Here's how the part is built. I have some questions about the finished solid (model axes, mm). A direction names the side the tool comes from. Give positions to 0.01 mm unless a question says otherwise; leave off trailing zeros. Order: outer loops, then holes, each group sorted by start corner. A loop starts at its lowest first (then second) coordinate and runs counter-clockwise, first axis right, second up. Notation, with made-up numbers: M -19,-2 L 35,-2 A15 ccw 35,24 Z; hole C 46,15 d7. An arc over 180 degrees is marked long. Use one line per item in the form item = value.
from build123d import *

# Parameters (mm, degrees)
F0_W        = 50.8
F0_H        = 50.8
F1_DEPTH    = 6.35
F3_DEPTH    = 9.144
F2_R        = 6.7603485979
F4_DEPTH    = 25.4
F5_R        = 5.08
F6_T1_DEPTH = 86.0732038629
F7_T        = 2.54
F7_T4_ANGLE = 49.6458001059
F7_T6_ANGLE = 79.2883730852


# Not quite as in the source:
# - a fillet or chamfer that OpenCascade refuses, or shapes differently, is made with other operations: its cross-section is extruded or revolved along the edge and cut away or added
# - a shell that OpenCascade refuses in one call is made with other operations: the cavity is built on its own and cut out


with BuildPart() as f1:
    # F0 (on Top) → F1 (new body)
    with BuildSketch(Plane.XY):
        with Locations((-25.4, 25.4)):
            Rectangle(F0_W, F0_H)
    extrude(amount=-F1_DEPTH)

    # F2 (on face) → F3 (join)
    with BuildSketch(Plane(origin=(0, 0, -6.35), x_dir=(1, 0, 0), z_dir=(0, 0, -1))):
        with BuildLine():
            ThreePointArc((0, 0), (-5.5886686099, -15.504363354), (-19.7841264307, -23.8773841411))
            ThreePointArc((-19.7841264307, -23.8773841411), (-12.8545439956, -39.5156757118), (0, -50.8))
            Line((0, -50.8), (0, 0))
        make_face()
    extrude(amount=F3_DEPTH)

    # F2 (on face) → F4 (cut)
    with BuildSketch(Plane(origin=(0, 0, -6.35), x_dir=(1, 0, 0), z_dir=(0, 0, -1))):
        with Locations((-37.9167422652, -20.3997846693)):
            Circle(F2_R)
    extrude(amount=-F4_DEPTH, mode=Mode.SUBTRACT)

    # F5
    f5_edges = [f1.edges().sort_by_distance(p)[0] for p in [
        (-50.8, 25.4, -6.35),
    ]]
    fillet(f5_edges, radius=F5_R)

    # F6: chamfer of 5.08 on 1 edges, made by hand

    # F6_s2 → F6_t1 (cut)
    with BuildSketch(Plane.XZ.offset(-63.8641495789)):
        Polygon((0, -10.414), (-5.08, -15.494), (0, -15.494), align=None)
    extrude(amount=F6_T1_DEPTH, mode=Mode.SUBTRACT)

    # F7: shell of thickness 2.54, made by hand


with BuildPart() as f7_core1:
    # F7_t2: copy of F1
    add(f1.part)

    # the walls: a layer under each face that stays
    f7_faces = [f7_core1.faces().sort_by_distance(p)[0] for p in [
        (-25.4, 0, -3.175),
        (-50.8, 25.4, -0.635),
        (-49.3121024484, 25.4, -4.8621024484),
        (-22.86, 25.4, -6.35),
        (0, 25.4, -5.207),
        (-25.4, 50.8, -3.175),
        (-44.6770908632, 20.3997846693, -3.175),
        (-12.8545439956, 39.5156757118, -10.922),
        (-5.5886686099, 15.504363354, -10.922),
        (-2.54, 25.4, -12.954),
        (-12.4320632154, 31.169630086, -15.494),
    ]]
    thicken(f7_faces, amount=-F7_T, mode=Mode.SUBTRACT)

    # F7_s3 → F7_t4 (revolve, cut)
    with BuildSketch(Plane(origin=(3.8753287702, 19.0692040386, 0), x_dir=(0, 0, 1), z_dir=(-0.1991535327, -0.9799683007, 0))):
        Polygon((-6.3754, 24.1684821625), (-3.81, 24.1430821625), (-3.81, 21.6030821625), (-6.35, 21.6030821625), align=None)
    revolve(axis=Axis((19.2103228569, 15.9527580845, -6.35), (0, 0, -1)), revolution_arc=F7_T4_ANGLE, mode=Mode.SUBTRACT)

    # F7_s5 → F7_t6 (revolve, cut)
    with BuildSketch(Plane.XZ):
        Polygon((-0.0254, -6.3754), (0, -3.81), (2.54, -3.81), (2.54, -6.35), align=None)
    revolve(axis=Axis((-24.3008235773, 0, -6.35), (0, 0, 1)), revolution_arc=F7_T6_ANGLE, mode=Mode.SUBTRACT)


with BuildPart() as f1_1:
    add(f1.part)

    # what is left inside the walls is the cavity
    f7_cavity = [f7_core1.part.solids().sort_by_distance(p)[0] for p in [
        (-25.4, 17.78, -0.0254),
    ]]
    add(f7_cavity, mode=Mode.SUBTRACT)


solid = f1_1.part
Q1. I want a section at C-C on z = -2.5. Write out the boundary of the cut face in (x, y).
Found:
outline = M -50.65,0 L 0,0 L 0,50.8 L -50.65,50.8 Z; C -37.92,20.4 d18.6; hole M -47.94,2.54 L -2.54,2.54 L -2.54,48.26 L -47.94,48.26 Z; hole C -37.92,20.4 d13.52
Q2. Thinking about a two-plate mould opening in Y: for faces 1 (the face through (-26, 50.8, -3)), 2 (the face through (-2.504, 31.4, -12.918)), 3 (the face through (-10, 31, -12.954)), which applies, +Y half, -Y half, draft (parallel to the pull), parting line (faces both ways), or undercut?
Found:
face_1 = +Y half
face_2 = draft
face_3 = undercut
Q3. I want a section at D-D on y = 39.5. Write out the boundary of the cut face in (x, z).
Found:
outline = M -50.8,-1.27 A5.08 ccw -45.72,-6.35 L -12.87,-6.35 L -12.87,-15.49 L -5.08,-15.49 L 0,-10.41 L 0,0 L -2.54,0 L -2.54,-9.36 L -6.13,-12.95 L -9.65,-12.95 L -9.65,-3.81 L -45.72,-3.81 A2.54 cw -48.26,-1.27 L -48.26,0 L -50.8,0 Z
Q4. I'm going to push flat-ended pins straight in: pin 1 Ø6 at (y, z) = (39.5, -13.5) entering from -X; pin 2 Ø2 at (y, z) = (12.5, -13.5) entering from +X; pin 3 Ø11 at (x, y) = (-37.92, 20.4) entering from +Z; pin 4 Ø13 at (x, y) = (-21, 29.5) entering from +Z. Where does each tip first touch, or does it pass through?
Found:
pin_1 = -14.87
pin_2 = -2.09
pin_3 = through
pin_4 = -3.81
Q5. I need wall thicknesses on L1, parallel to Y at x = -4.5, z = -0.75; L2, parallel to X at y = 6, z = -1; L3, parallel to Y at x = -30.5, z = -3. Which ranges of each line are inside material? Lowest first, please.
Found:
L1 = 0 to 2.54, 48.26 to 50.8
L2 = -50.8 to -48.26, -2.54 to 0
L3 = 0 to 2.54, 14.79 to 26.01, 48.26 to 50.8
Q6. I want a section at B-B on x = -24. Write out the boundary of the cut face in (y, z).
Found:
outline = M 0,-6.35 L 50.8,-6.35 L 50.8,0 L 48.26,0 L 48.26,-3.81 L 2.54,-3.81 L 2.54,0 L 0,0 Z
Q7. I want a section at A-A on z = -7.75. Write out the boundary of the cut face in (x, y).
Found:
outline = M -19.78,23.88 A24.3 cw 0,0 L 0,50.8 A39.79 ccw Z; hole M -16.73,25.75 A26.84 cw -2.54,15.71 L -2.54,46.2 A37.25 ccw Z
Q8. On a 3-axis mill with a long thin cutter (end or side, diameter ignored), from which of +Z, -Z, +X, -X, +Y, -Y can I reach the whole of each face in a straight line? I mean faces 4 (the face through (-24, 26, -3.81)), 5 (the face through (-26, 0, -3)), 6 (the face through (-12.997, 39.321, -10.858)). Say none if no direction works.
Found:
face_4 = +Z
face_5 = +Z, -Z, +X, -X, -Y
face_6 = -Z, -X, +Y
